Design review of the part built by this model. Coordinates are the model's own, in mm. Face numbers are marked on the shaded views. A direction names the side the tool comes from. Round coordinates to 2 decimals unless told otherwise and drop trailing zeros. Write each loop counter-clockwise with the first axis right and the second up, starting at its lowest first coordinate (ties: lowest second). Pieces come first, ordered by that corner, then holes. Notation, with made-up numbers: (43, 34.5) -> (86, 34.5) arc R17 cw to (86, 41.5) -> close; hole circle Ø1 at (81.5, 79.25). An arc over 180 degrees is marked (long way). One line per question, with ' | ' between items. Start each with the question number.
1) Insertion check: pin 1 Ø1 at (y, z) = (32, -5) entering from -X; pin 2 Ø3 at (y, z) = (33, -4.5) entering from +X. Each pin has a flat end and moves straight along its axis. Give the tip position at first contact, or say it passes through.
2) Consider section B-B (y = 49). Give the boundary of the cut face in (x, z).
3) For the marked faces 4, 5 and 6, list the 3-axis set-ups (+Z, -Z, +X, -X, +Y, -Y) from which the entire face can be reached by the end or side of a thin tool; tool diameter is ignored.
4) Consider section A-A (z = -5.25). Give the boundary of the cut face in (x, y).
5) Consider section D-D (y = 26.5). Give the boundary of the cut face in (x, z).
6) For probe 1 along X at (y, z) = (23, -2.5); probe 2 along Y at (x, z) = (-8, -0.75); probe 3 along Y at (x, z) = (7.5, -5), list the stretches that pass through material, from the lowest coordinate up.
7) Consider section C-C (x = -29). Give the boundary of the cut face in (y, z).
8) Mouldability with a two-part tool opening along Y and no side actions: class the marked faces 1, 2 and 3 as +Y half, -Y half, draft (parallel to the pull), parting line (faces both ways), or undercut.
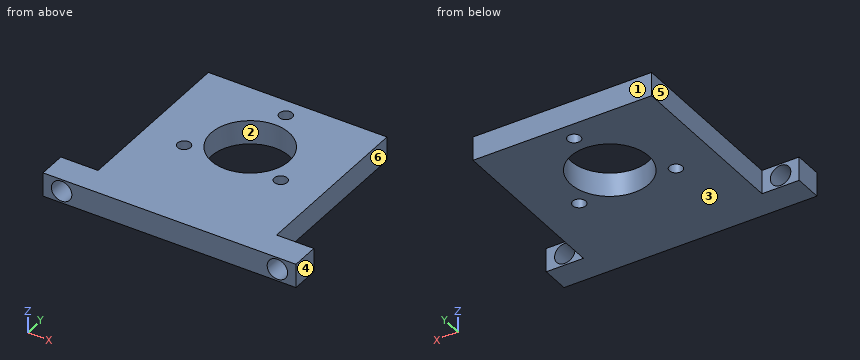
```python
from build123d import *

# Parameters (mm, degrees)
SKETCH2_R                  = 4.175
BOSS_EXTRUDE1_DEPTH        = 6.4
SKETCH3_R                  = 10.5
CUT_EXTRUDE1_DEPTH         = 65.132363125
F_3_5_3_5_DIAMETER_HOLE1_D = 3.5
CIRPATTERN1_COUNT          = 3
CUT_EXTRUDE2_DEPTH         = 58.958692187
CUT_EXTRUDE2_DEPTH_BACK    = 58.958692187
SKETCH12_R                 = 2.75


with BuildPart() as part:
    # Sketch2 → Boss-Extrude1 (new body)
    with BuildSketch(Plane.XY):
        Polygon((-34, 0), (34, 0), (34, 7.5), (24, 7.5), (24, 54), (-24, 54), (-24, 7.5), (-34, 7.5), align=None)
        with Locations((0, 34)):
            Circle(SKETCH2_R, mode=Mode.SUBTRACT)
    extrude(amount=-BOSS_EXTRUDE1_DEPTH)

    # Sketch3 → Cut-Extrude1 (cut, through all)
    with BuildSketch(Plane(origin=(0, 0, -6.4), x_dir=(-1, 0, 0), z_dir=(0, 0, -1))):
        with Locations((0, 34)):
            Circle(SKETCH3_R)
    extrude(amount=-CUT_EXTRUDE1_DEPTH, mode=Mode.SUBTRACT)

    # Ø3.5 (3.5) Diameter Hole1 (through all)
    with Locations(Plane.XY):
        with Locations((0, 49)):
            f_3_5_3_5_diameter_hole1 = Hole(F_3_5_3_5_DIAMETER_HOLE1_D / 2)

    # CirPattern1: Ø3.5 (3.5) Diameter Hole1 ×3 about axis
    cirpattern1_axis = Axis((0, 34, 0), (0, 0, 1))
    for i in range(1, CIRPATTERN1_COUNT):
        add(f_3_5_3_5_diameter_hole1.rotate(cirpattern1_axis, i * 360 / CIRPATTERN1_COUNT), mode=Mode.SUBTRACT)

    # Sketch12 → Cut-Extrude2 (cut, two sides: drawn at the far end of the back side and taken through both)
    with BuildSketch(Plane(origin=(0, 7.5, 0), x_dir=(1, 0, 0), z_dir=(0, 1, 0)).offset(-CUT_EXTRUDE2_DEPTH_BACK)):
        with Locations(Location((-29, 3.2, 0), (0, 0, 90))):
            Circle(SKETCH12_R)
        with Locations(Location((29, 3.2, 0), (0, 0, 90))):
            Circle(SKETCH12_R)
    extrude(amount=CUT_EXTRUDE2_DEPTH + CUT_EXTRUDE2_DEPTH_BACK, mode=Mode.SUBTRACT)


solid = part.part
```
From the geometry:
1) pin 1: stops at x = -24 | pin 2: stops at x = 24
2) outline: (-24, -6.4) -> (-1.75, -6.4) -> (-1.75, 0) -> (-24, 0) -> close; (1.75, -6.4) -> (24, -6.4) -> (24, 0) -> (1.75, 0) -> close
3) face 4: +Z, -Z, +X, +Y, -Y | face 5: +Z, -Z, -X, +Y | face 6: +Z, -Z, +X, +Y
4) outline: (-34, 0) -> (-30.83, 0) -> (-30.83, 7.5) -> (-34, 7.5) -> close; (-27.17, 0) -> (27.17, 0) -> (27.17, 7.5) -> (24, 7.5) -> (24, 54) -> (-24, 54) -> (-24, 7.5) -> (-27.17, 7.5) -> close; (30.83, 0) -> (34, 0) -> (34, 7.5) -> (30.83, 7.5) -> close; hole circle Ø3.5 at (-12.99, 26.5); hole circle Ø21 at (0, 34); hole circle Ø3.5 at (0, 49); hole circle Ø3.5 at (12.99, 26.5)
5) outline: (-24, -6.4) -> (-14.74, -6.4) -> (-14.74, 0) -> (-24, 0) -> close; (-11.24, -6.4) -> (-7.35, -6.4) -> (-7.35, 0) -> (-11.24, 0) -> close; (7.35, -6.4) -> (11.24, -6.4) -> (11.24, 0) -> (7.35, 0) -> close; (14.74, -6.4) -> (24, -6.4) -> (24, 0) -> (14.74, 0) -> close
6) probe 1: x = -24 to 24 | probe 2: y = 0 to 27.2, 40.8 to 54 | probe 3: y = 0 to 26.65, 41.35 to 54
7) outline: (0, -6.4) -> (7.5, -6.4) -> (7.5, -5.95) -> (0, -5.95) -> close; (0, -0.45) -> (7.5, -0.45) -> (7.5, 0) -> (0, 0) -> close
8) face 1: +Y half | face 2: undercut | face 3: draft
